The drawing under review shows one solid part. Ordinate dimensions are in mm from its lowest x, y, z. A direction names the side the tool comes from. Round coordinates to 2 decimals unless told otherwise and drop trailing zeros. Order: outer loops, then holes, each group sorted by start corner. A loop starts at its lowest first (then second) coordinate and runs counter-clockwise, first axis right, second up. Notation, with made-up numbers: M -3.75,84 L 21.25,84 A27 cw 21.25,116 Z; hole C -30,50 d9. An arc over 180 degrees is marked long. Answer as a JSON object with one key per item and string values.
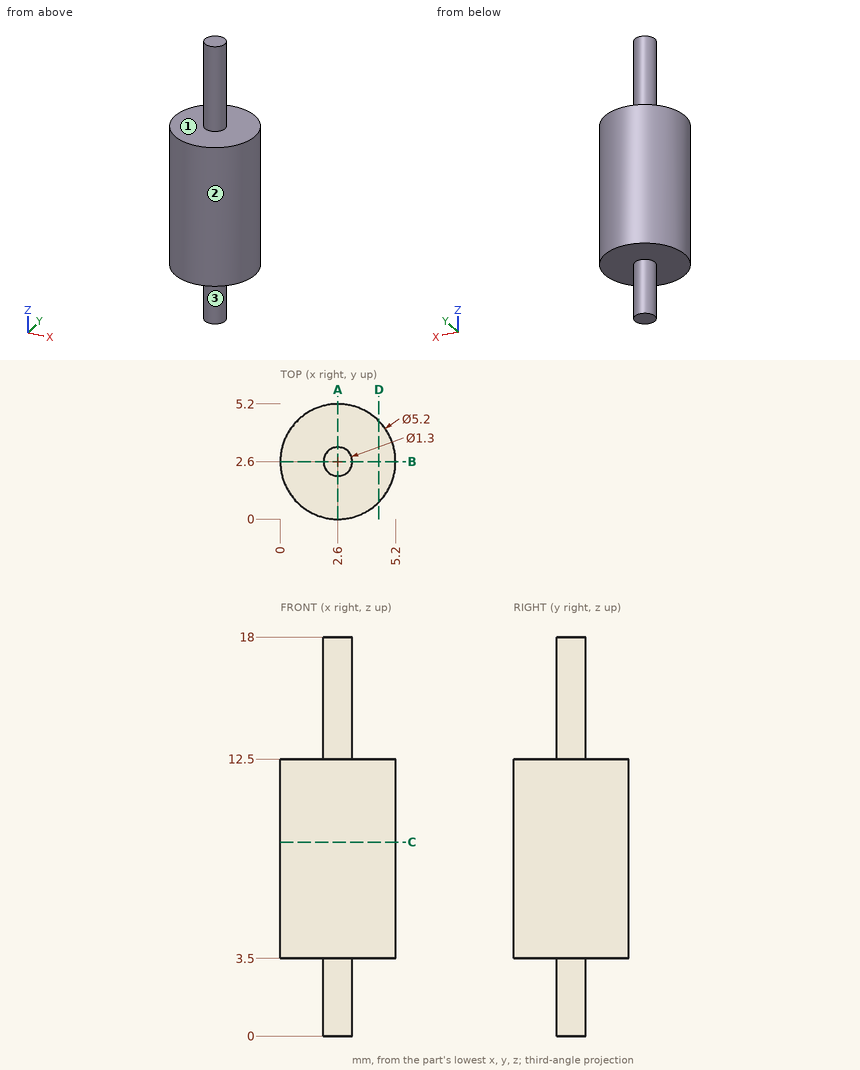
1) Add section D-D on x = 4.45. State the section outline as (y, z) points, and give its area (3 significant figures).
Geometry check:
{"outline": "M 0.77,3.5 L 4.43,3.5 L 4.43,12.5 L 0.77,12.5 Z", "area": "32.9 mm²"}
2) Insertion check: P1, Ø1, axis at x = 4, z = 3.5, coming from the -Y side; P2, Ø1.6, axis at x = 2, y = 4, coming from the -Z side; P3, Ø2, axis at x = 3, z = 11, coming from the -Y side; P4, Ø1, axis at y = 2, z = 14.5, coming from the -X side. Each pin has a flat end and moves straight along its axis. Give the tip position at first contact, or say it passes through.
Geometry check:
{"P1": "stops at y = 0.16", "P2": "stops at z = 3.5", "P3": "stops at y = 0", "P4": "stops at x = 1.96"}
3) Machinability: for the marked faces 1, 2 and 3, which of the approach directions +Z, -Z, +X, -X, +Y, -Y give a long, thin tool a straight path to every point of the face, cutting with its end or side? Answer none if there is none.
Geometry check:
{"face 1": "+Z", "face 2": "+Z, -Z", "face 3": "-Z"}
4) Add section C-C on z = 8.75. State the section outline as (x, y) points, and give its area (3 significant figures).
Geometry check:
{"outline": "C 2.6,2.6 d5.2", "area": "21.2 mm²"}
5) For L1, parallel to Z at x = 3.3, y = 1.6; L2, parallel to Y at x = 0.35, z = 7; L3, parallel to X at y = 1.3, z = 5.5, list the stretches that pass through material, from the lowest coordinate up.
Geometry check:
{"L1": "z = 3.5 to 12.5", "L2": "y = 1.3 to 3.9", "L3": "x = 0.35 to 4.85"}
6) Add section A-A on x = 2.6. State the section outline as (y, z) points, and give its area (3 significant figures).
Geometry check:
{"outline": "M 0,3.5 L 1.95,3.5 L 1.95,0 L 3.25,0 L 3.25,3.5 L 5.2,3.5 L 5.2,12.5 L 3.25,12.5 L 3.25,18 L 1.95,18 L 1.95,12.5 L 0,12.5 Z", "area": "58.5 mm²"}
